Autodesk Inventor part; units mm, degrees
ref_plane "YZ Plane" through (0, 0, 0) normal (1, 0, 0) x (0, 1, 0)
ref_plane "XZ Plane" through (0, 0, 0) normal (0, 1, 0) x (-1, 0, 0)
ref_plane "XY Plane" through (0, 0, 0) normal (0, 0, 1) x (1, 0, 0)
sketch "Szkic1" plane through (0, 0, 0) normal (0, 0, 1) x (1, 0, 0)
  line L0 (-215, -55) -> (215, -55) construction
  line L1 (215, -55) -> (215, 55) construction
  line L2 (215, 55) -> (-215, 55) construction
  line L3 (-215, 55) -> (-215, -55) construction
  line L4 (-215, -55) -> (215, 55) construction
  line L5 (215, -55) -> (-215, 55) construction
  circle A0 centre (-280, 8) radius 41.25 construction
  circle A1 centre (-280, 8) radius 11
  arc A2 (-280, 33) -> (-296.3719, -10.8934) centre (-280, 8) ccw
  line L6 (-280, 33) -> (-111.2284, 33)
  line L7 (-236.8172, -62.5) -> (215, -62.5)
  line L8 (-296.3719, -10.8934) -> (-236.8172, -62.5)
  arc A3 (-296.3719, -10.8934) -> (-280, 33) centre (-280, 8) ccw construction
  circle A4 centre (-200, -120) radius 25 construction
  circle A5 centre (-120, -120) radius 25 construction
  circle A6 centre (-40, -120) radius 25 construction
  circle A7 centre (40, -120) radius 25 construction
  circle A8 centre (120, -120) radius 25 construction
  circle A9 centre (200, -120) radius 25 construction
  line L9 (-120, -120) -> (-40, -120) construction
  line L10 (40, -120) -> (120, -120) construction
  arc A10 (-111.2284, 33) -> (-96.7716, 33) centre (-104, 31) ccw construction
  arc A11 (96.7716, 33) -> (111.2284, 33) centre (104, 31) ccw construction
  line L11 (-96.7716, 33) -> (96.7716, 33)
  line L12 (-111.2284, 33) -> (-96.7716, 33) construction
  arc A12 (-96.7716, 33) -> (-111.2284, 33) centre (-104, 31) ccw
  arc A13 (111.2284, 33) -> (96.7716, 33) centre (104, 31) ccw
  line L13 (111.2284, 33) -> (233.5, 33)
  line L14 (96.7716, 33) -> (111.2284, 33) construction
  arc A14 (240.9621, 24.7471) -> (233.5, 33) centre (233.5, 25.5) ccw
  arc A15 (231.7135, -47.4781) -> (234.1621, -42.6529) centre (226.7, -41.9) ccw
  line L15 (240.9621, 24.7471) -> (234.1621, -42.6529)
  arc A16 (233.5, 33) -> (240.9621, 24.7471) centre (233.5, 25.5) ccw construction
  line L16 (215, -62.5) -> (231.7135, -47.4781)
  arc A17 (234.1621, -42.6529) -> (231.7135, -47.4781) centre (226.7, -41.9) ccw construction
  point P0 (0, 0)
  point P1 (-215, 25.5)
  point P2 (-215, -44.5)
  point P3 (215, 25.5)
  point P4 (215, -44.5)
  point P5 (-252.055, -39.3717)
  point P6 (-80, -120)
  point P7 (80, -120)
  point P8 (-150, -32.735)
  point P9 (-20, -50)
  point P10 (20, -50)
  point P11 (140, -55)
  point P12 (-178.648, -14.42)
  point P13 (160.115, -11.966)
  point P14 (-40.115, -6.966)
  point P15 (40.115, -6.966)
  point P16 (0, -55)
  point P17 (-160, -55)
  point P18 (160, -55)
  point P19 (-154.542, 27.216)
  point P20 (-7.339, 11.921)
  point P21 (7.339, 11.921)
  point P22 (127.339, 6.921)
  dimension "d0" = 430
  dimension "d1" = 110
  dimension "d2" = 63
  dimension "d3" = 65
  dimension "d4" = 82.5
  dimension "d7" = 22
  dimension "d8" = 50
  dimension "d9" = 17.5
  dimension "d10" = 70
  dimension "d11" = 7.5
  dimension "d12" = 7.5
  dimension "d13" = 7.5
  dimension "d15" = 55
  dimension "d16" = 15
  dimension "d17" = 50
  dimension "d18" = 65
  dimension "d21" = 80
  dimension "d26" = 23
  dimension "d27" = 208
  dimension "d28" = 104
  dimension "d29" = 15
  dimension "d30" = 15
  dimension "d31" = 18.5
  dimension "d32" = 67.4
  dimension "d33" = 6.8
  dimension "d34" = 15
  dimension "d35" = 15
  dimension "d38" = 70
  dimension "d39" = 60
  dimension "d40" = 60
  dimension "d41" = 60
  dimension "d43" = 18.315
  dimension "d44" = 39.885
  dimension "d45" = 43.034
  dimension "d46" = 39.885
  dimension "d47" = 39.885
  dimension "d48" = 40
  dimension "d49" = 40
  dimension "d50" = 59.951
  dimension "d52" = 61.921
  dimension "d53" = 12.661
  dimension "d54" = 12.661
  dimension "d55" = 12.661
  dimension "d56" = 61.921
  dimension "d73" = 130
  dimension "d74" = 40.735
  dimension "d75" = 28.648
  dimension "d76" = 4.542
  dimension "d77" = 43.034
extrude "Wyciągnięcie proste1" add sketch "Szkic1" along normal blind 5
hole "Otwór1" at (-280, 8, 0) at (-215, 25.5, 0) at (-215, -44.5, 0) at (215, 25.5, 0) at (215, -44.5, 0) at (-252.055, -39.3717, 0) at (-200, -120, 0) at (-120, -120, 0) at (-40, -120, 0) at (40, -120, 0) at (120, -120, 0) at (200, -120, 0) at (-80, -120, 0) at (80, -120, 0) at (-104, 31, 0) at (104, 31, 0) at (226.7, -41.9, 0) at (0, -55, 0) at (-160, -55, 0) at (160, -55, 0) at (-154.542, 27.216, 0) at (-7.339, 11.921, 0) at (7.339, 11.921, 0) at (127.339, 6.921, 0) direction (0, 0, 1) diameter 5 end through all
hole "Otwór2" at (233.5, 25.5, 0) at (-150, -32.735, 0) at (-20, -50, 0) at (20, -50, 0) at (140, -55, 0) at (-178.648, -14.42, 0) at (160.115, -11.966, 0) at (-40.115, -6.966, 0) at (40.115, -6.966, 0) direction (0, 0, 1) diameter 6 end through all
equation "\"d12\" = d11"
equation "\"d29\" = 2 * d11"
equation "\"d30\" = d29"
equation "\"d34\" = d30"
equation "\"d35\" = d34"
properties part number "plyta_boczna"
The listing builds one solid part. Answer for the finished solid, in the listing's coordinates (mm). Give positions to 0.01 mm unless a question says otherwise; leave off trailing zeros. Loops run counter-clockwise (first coordinate to the right, second up) from the corner with the lowest first, then second, coordinate; pieces in that order, holes last. Notation, with made-up numbers: (77.5, -36.5) - (101.5, -36.5) arc R14 ccw to (101.5, -28.5) - close; hole circle Ø1 at (1.5, -15.5). An arc over 180 degrees is marked (long way). Write each question's results on one line, items separated by ' | '.
1. Find section A-A, the plane x = 195. Write down the section's boundary in (y, z), then the cut area to 4 significant figures.
Resolved:
outline: (-62.5, 0) - (33, 0) - (33, 5) - (-62.5, 5) - close | area: 477.5 mm^2
2. Flat-ended cylindrical pins translate along their axes: P1, Ø2.5, axis at x = -199.5, z = 2.5, coming from the +Y side; P2, Ø2, axis at y = -34, z = 2.5, coming from the +X side. Find the tip coordinate at first contact, or state that the pin passes through.
Resolved:
P1: stops at y = 33 | P2: stops at x = 235.14
3. For a pull along X with two mould halves and no side action, classify faces 1 (the face through (-303.569, 16.338, 2.465)), 2 (the face through (-36, -11, 0)), 3 (the face through (-291, 8, 2)), 4 (the face through (223.24, -55.094, 2.465)) as +X half, -X half, draft (parallel to the pull), parting line (faces both ways), or undercut.
Resolved:
face 1: -X half | face 2: draft | face 3: undercut | face 4: +X half
4. Find section B-B, the plane z = 1.45. Count the separate pieces of the cut face and the enclosed holes in it, then the cut area to 3 significant figures.
Resolved:
separate pieces: 1 | enclosed holes: 25 | area: 48,600 mm^2
5. Consider probe 1 along Y at (x, z) = (-215, 1.75); probe 2 along X at (y, z) = (-13.5, 1.4); probe 3 along Y at (x, z) = (-20, 2.95). Determine where each line is inside the solid, lowest interval first. Write a range as from..to.
Resolved:
probe 1: y = -62.5..-47, -42..23, 28..33 | probe 2: x = -293.36..-181.5, -175.79..157.54, 162.69..237.1 | probe 3: y = -62.5..-53, -47..33
